Check sheet for the modelled part. Datum: model origin and axes. Units: mm. A direction names the side the tool comes from. Coordinates: 2 decimals unless noted, no trailing zeros. Write each loop counter-clockwise with the first axis right and the second up, starting at its lowest first coordinate (ties: lowest second). Pieces come first, ordered by that corner, then holes. Notation, with made-up numbers: (26, 81.25) -> (80, 81.25) arc R30 ccw to (80, 109.25) -> close; hole circle Ø2 at (73, 29.5). An arc over 180 degrees is marked (long way). Put each result on its own line as item: value.
```python
from build123d import *

# Parameters (mm, degrees)
F1_DEPTH = 127
F3_DEPTH = 5.842
F5_W     = 21.162301302
F5_H     = 28.62467058
F5_W_2   = 8.4839835763
F5_W_3   = 10.6764808297
F5_W_4   = 10.2951750159
F5_W_5   = 9.0689621866
F5_W_6   = 20.9719697013
F6_DEPTH = 6.604
F7_W     = 50.9557463229
F7_H     = 29.4899502769
F8_DEPTH = 2.54


with BuildPart() as f1:
    # F0 (on Front) → F1 (new body)
    with BuildSketch(Plane.XZ):
        Polygon((46.8764491379, 81.9781199098), (-47.2529642284, 0), (-39.5179688628, 0), (-8.6630821907, 26.8717875629), (-8.6630821907, 0), (-3.5830821907, 0), (-3.5830821907, 31.2960034828), (41.7964491379, 70.817429652), (41.7964491379, 0), (46.8764491379, 0), align=None)
    extrude(amount=F1_DEPTH)

    # F2 (on face) → F3 (cut)
    with BuildSketch(Plane.YZ.offset(46.8764491379)):
        Polygon((-50.4709516168, 40.3369802166), (-58.757108451, 35.0823956511), (-50.4709516168, 29.8278110855), align=None)
        Polygon((-35.8090658188, 49.6346703711), (-44.928032577, 43.8519676127), (-44.928032577, 26.3128236894), (-35.8090658188, 20.530120931), align=None)
        Polygon((-30.3332541585, 17.0576890172), (-8.9731920958, 3.5124165006), (-8.9731920958, 66.6523748015), (-30.3332541585, 53.107102285), align=None)
        Polygon((-30.3332541585, 0), (-12.9201102982, 0), (-30.3332541585, 11.0423732976), align=None)
        Polygon((-44.928032577, 0), (-35.8090658188, 0), (-35.8090658188, 14.5148052115), (-44.928032577, 20.2975079699), align=None)
        Polygon((-61.4131574035, 30.7513871575), (-61.4131574035, 0), (-50.4709516168, 0), (-50.4709516168, 23.812495366), align=None)
        Polygon((-76.5290483832, 23.812495366), (-76.5290483832, 0), (-65.5868425965, 0), (-65.5868425965, 30.7513871575), align=None)
        Polygon((-91.1909341812, 14.5148052115), (-91.1909341812, 0), (-82.071967423, 0), (-82.071967423, 20.2975079699), align=None)
        Polygon((-96.6667458415, 11.0423732976), (-114.0798897018, 0), (-96.6667458415, 0), align=None)
        Polygon((-118.0268079042, 66.6523748015), (-118.0268079042, 3.5124165006), (-96.6667458415, 17.0576890172), (-96.6667458415, 53.107102285), align=None)
        Polygon((-82.071967423, 43.8519676127), (-91.1909341812, 49.6346703711), (-91.1909341812, 20.530120931), (-82.071967423, 26.3128236894), align=None)
        Polygon((-68.242891549, 35.0823956511), (-76.5290483832, 40.3369802166), (-76.5290483832, 29.8278110855), align=None)
        Polygon((-65.5868425965, 39.4134041447), (-65.5868425965, 72.1255466342), (-76.5290483832, 72.1255466342), (-76.5290483832, 46.3522959362), align=None)
        Polygon((-96.6667458415, 72.0583349466), (-117.0658916235, 72.0583349466), (-96.6667458415, 59.1224180045), align=None)
        Polygon((-82.071967423, 72.1255466342), (-91.1909341812, 72.1255466342), (-91.1909341812, 55.6499860907), (-82.071967423, 49.8672833323), align=None)
        Polygon((-50.4709516168, 72.1255466342), (-61.4131574035, 72.1255466342), (-61.4131574035, 39.4134041447), (-50.4709516168, 46.3522959362), align=None)
        Polygon((-35.8090658188, 72.1255466342), (-44.928032577, 72.1255466342), (-44.928032577, 49.8672833323), (-35.8090658188, 55.6499860907), align=None)
        Polygon((-30.3332541585, 59.1224180045), (-9.9341083765, 72.0583349466), (-30.3332541585, 72.0583349466), align=None)
    extrude(amount=-F3_DEPTH, mode=Mode.SUBTRACT)

    # F5 (on face) → F6 (cut)
    with BuildSketch(Plane.YZ.offset(-3.5830821907)):
        with Locations((-107.3864251375, 14.31233529)):
            Rectangle(F5_W, F5_H)
        with Locations((-86.4624343812, 14.31233529)):
            Rectangle(F5_W_2, F5_H)
        with Locations((-70.972006768, 14.31233529)):
            Rectangle(F5_W_3, F5_H)
        with Locations((-55.8152236044, 14.31233529)):
            Rectangle(F5_W_4, F5_H)
        with Locations((-40.2838084847, 14.31233529)):
            Rectangle(F5_W_5, F5_H)
        with Locations((-19.5952425711, 14.31233529)):
            Rectangle(F5_W_6, F5_H)
    extrude(amount=-F6_DEPTH, mode=Mode.SUBTRACT)

    # F7 (on face) → F8 (join)
    with BuildSketch(Plane(origin=(-20.3815104704, 0, 23.4025813987), x_dir=(0.7541036669, 0, 0.6567554032), z_dir=(-0.6567554032, 0, 0.7541036669))):
        with Locations((58.2807790488, -20.9741364233)):
            Rectangle(F7_W, F7_H)
        Polygon((83.7586522102, -63.5), (83.7586522102, -46.6593503952), (32.8029058874, -46.6593503952), (32.8029058874, -63.5), (32.8029058874, -80.3406496048), (83.7586522102, -80.3406496048), align=None)
        with Locations((58.2807790488, -106.0258635767)):
            Rectangle(F7_W, F7_H)
        with Locations((-4.7251372654, -106.0258635767)):
            Rectangle(F7_W, F7_H)
        Polygon((-30.2030104268, -46.6593503952), (-30.2030104268, -63.5), (-30.2030104268, -80.3406496048), (20.752735896, -80.3406496048), (20.752735896, -63.5), (20.752735896, -46.6593503952), align=None)
        with Locations((-4.7251372654, -20.9741364233)):
            Rectangle(F7_W, F7_H)
    extrude(amount=F8_DEPTH)


solid = f1.part
```
Q1. Tool access check on faces 3 (the flat face through (-8.663, -94, 14)), 4 (the flat face through (-6, -44.818, 14)), 5 (the flat face through (44.372, -19.504, 59.975)), 6 (the flat face through (23, -46.659, 63)), 7 (the flat face through (-25.88, -63.26, 21.98)). Record the directions out of +Z, -Z, +X, -X, +Y, -Y that give a thin tool (end or side, any length) a straight path to the whole face; none if there is none.
Recorded:
face 3: -Z, +Y, -Y
face 4: -Z
face 5: +X
face 6: +Z, -X
face 7: +Z, -X, +Y, -Y
Q2. Mould release check, pull along Y, two halves, no side actions. Record for faces 1 (the flat face through (-25, -80.341, 21)), 2 (the flat face through (21.63, -20.77, 63.36)): released by +Y, released by -Y, zero draft, split by the parting line, or undercut.
Recorded:
face 1: undercut
face 2: zero draft
Q3. Cross-section at B-B (x = 10.5). Record the cut outline in (y, z).
Recorded:
outline: (-127, 43.56) -> (0, 43.56) -> (0, 50.3) -> (-6.23, 50.3) -> (-6.23, 53.67) -> (-35.72, 53.67) -> (-35.72, 50.3) -> (-46.66, 50.3) -> (-46.66, 53.67) -> (-80.34, 53.67) -> (-80.34, 50.3) -> (-91.28, 50.3) -> (-91.28, 53.67) -> (-120.77, 53.67) -> (-120.77, 50.3) -> (-127, 50.3) -> close
Q4. Depth check by flat-ended pin: P1, Ø6.5, axis at y = -95, z = 18, coming from the -X side; P2, Ø12, axis at y = -97.5, z = 45, coming from the -X side; P3, Ø4, axis at x = -13, y = -54, coming from the -Z side. Enter the tip coordinate at first touch or a pass-through.
Recorded:
P1: stops at x = -34.18
P2: stops at x = -2.47
P3: stops at z = 21.35
Q5. Cross-section at A-A (y = -78.5). Record the cut outline in (x, z), plus the area to 3 significant figures.
Recorded:
outline: (-47.25, 0) -> (-39.52, 0) -> (-8.66, 26.87) -> (-8.66, 0) -> (-3.58, 0) -> (-3.58, 31.3) -> (41.8, 70.82) -> (41.8, 0) -> (46.88, 0) -> (46.88, 81.98) -> (42.78, 78.41) -> (41.11, 80.33) -> (2.69, 46.86) -> (4.36, 44.95) -> (-4.73, 37.03) -> (-6.4, 38.95) -> (-44.83, 5.48) -> (-43.16, 3.57) -> close
area: 1,390 mm2
Q6. Material ranges on line 1 along X through (y, z) = (-65, 25); line 2 along X through (y, z) = (-108, 78.5); line 3 along X through (y, z) = (-31.5, 6.5), recorded low to high.
Recorded:
line 1: x = -22.41 to -10.81, -8.66 to -3.58, 41.8 to 46.88
line 2: x = 39.02 to 42.7, 42.88 to 46.88
line 3: x = -43.66 to -32.05, -8.66 to -3.58, 41.8 to 46.88
Q7. Cross-section at D-D (z = 51.5). State how many separate pieces and enclosed holes the cut face has, plus the area to 3 significant figures.
Recorded:
separate pieces: 8
enclosed holes: 0
area: 1,630 mm2
Q8. Cross-section at C-C (y = -108.5). Record the cut outline in (x, z), plus the area to 3 significant figures.
Recorded:
outline: (-47.25, 0) -> (-39.52, 0) -> (-10.19, 25.54) -> (-10.19, 28.62) -> (-3.58, 28.62) -> (-3.58, 31.3) -> (41.03, 70.15) -> (41.03, 72.06) -> (46.88, 72.06) -> (46.88, 81.98) -> (42.78, 78.41) -> (41.11, 80.33) -> (2.69, 46.86) -> (4.36, 44.95) -> (-4.73, 37.03) -> (-6.4, 38.95) -> (-44.83, 5.48) -> (-43.16, 3.57) -> close; (41.8, 3.54) -> (46.88, 3.54) -> (46.88, 9.55) -> (41.8, 9.55) -> close; (41.8, 60.61) -> (46.88, 60.61) -> (46.88, 66.63) -> (41.8, 66.63) -> close
area: 930 mm2
